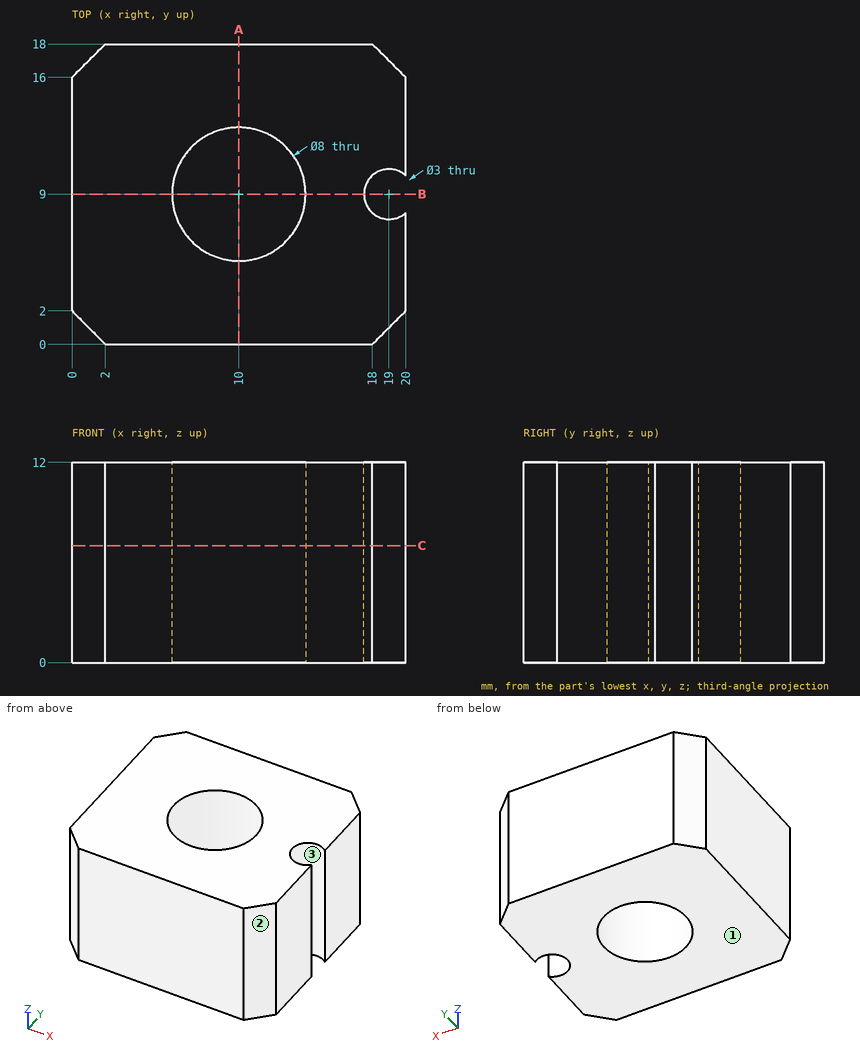
Answer from the drawing. Dimensions are ordinates in mm from the lowest x, y and z of the part. Give positions to 0.01 mm unless a question says otherwise; leave off trailing zeros. Write each loop counter-clockwise with the first axis right and the second up, starting at its lowest first coordinate (ties: lowest second). Pieces come first, ordered by that corner, then holes. Notation, with made-up numbers: (61.5, 42.25) - (79.5, 42.25) arc R19 cw to (79.5, 77.25) - close; hole circle Ø1 at (77.25, 70). An arc over 180 degrees is marked (long way). Answer in a Markdown table with one row per item. Add a question column.
Item 1: Section C-C, the plane z = 7 is taken. Write down the section's boundary in (x, y), and give its area (3 significant figures).
Item 2: Section B-B, the plane y = 9 is taken. Write down the section's boundary in (x, z), and give its area (3 significant figures).
Item 3: Find the intervals of material crossed by L1, parallel to Y at x = 10, z = 8; L2, parallel to Y at x = 19, z = 4; L3, parallel to X at y = 7, z = 1.5, in increasing order.
Item 4: A flat-ended cylindrical pin translates along its axis: P1, Ø7, axis at x = 10, y = 9, coming from the -Z side. Find the tip coordinate at first contact, or state that the pin passes through.
Item 5: Determine the mould class of the marked faces 1, 2 and 3 for opening direction Y: pulls with the +Y half, pulls with the -Y half, needs draft (parallel to the pull), parting line crosses it, or undercut.
Item 6: Section A-A, the plane x = 10 is taken. Write down the section's boundary in (y, z), and give its area (3 significant figures).
Recorded:
| question | item | result |
|---|---|---|
| 1 | outline | (0, 2) - (2, 0) - (18, 0) - (20, 2) - (20, 7.88) arc R1.5 cw (long way) to (20, 10.12) - (20, 16) - (18, 18) - (2, 18) - (0, 16) - close; hole circle Ø8 at (10, 9) |
| 1 | area | 295 mm2 |
| 2 | outline | (0, 0) - (6, 0) - (6, 12) - (0, 12) - close; (14, 0) - (17.5, 0) - (17.5, 12) - (14, 12) - close |
| 2 | area | 114 mm2 |
| 3 | L1 | y = 0 to 5, 13 to 18 |
| 3 | L2 | y = 1 to 7.5, 10.5 to 17 |
| 3 | L3 | x = 0 to 6.54, 13.46 to 20 |
| 4 | P1 | passes through |
| 5 | face 1 | needs draft |
| 5 | face 2 | pulls with the -Y half |
| 5 | face 3 | undercut |
| 6 | outline | (0, 0) - (5, 0) - (5, 12) - (0, 12) - close; (13, 0) - (18, 0) - (18, 12) - (13, 12) - close |
| 6 | area | 120 mm2 |
